```python
from build123d import *

# Parameters (mm, degrees)
EXTRUDE_1_DEPTH             = 2
EXTRUDE_2_REACH             = 86.23
EXTRUDE_2_DIRECTION_2_REACH = 86.23
CUT_EXTRUDE_2_DEPTH         = 114.341574455
FILLET_2_R                  = 1
SKETCH_8_R                  = 1.6
CUT_EXTRUDE_3_DEPTH         = 121.450189292
SKETCH_10_R                 = 1.6
SKETCH_10_W                 = 3.5
SKETCH_10_H                 = 20
CUT_EXTRUDE_5_DEPTH         = 86.056598939
SKETCH_11_R                 = 8.05
SKETCH_11_R_2               = 6.05
CUT_EXTRUDE_6_DEPTH         = 86.056598939
SKETCH_12_W                 = 25
SKETCH_12_H                 = 25
CUT_EXTRUDE_7_DEPTH         = 86.056598939
FILLET_3_R                  = 1


with BuildPart() as part:
    # 草图1 → 凸台-拉伸1 (new body)
    with BuildSketch(Plane.XY):
        with BuildLine():
            Line((72.25, -38.25), (72.25, 38.25))
            ThreePointArc((72.25, 38.25), (70.785533906, 41.785533906), (67.25, 43.25))
            Line((67.25, 43.25), (-67.25, 43.25))
            ThreePointArc((-67.25, 43.25), (-70.785533906, 41.785533906), (-72.25, 38.25))
            Line((-72.25, 38.25), (-72.25, -38.25))
            ThreePointArc((-72.25, -38.25), (-70.785533906, -41.785533906), (-67.25, -43.25))
            Line((-67.25, -43.25), (67.25, -43.25))
            ThreePointArc((67.25, -43.25), (70.785533906, -41.785533906), (72.25, -38.25))
        make_face()
    extrude(amount=EXTRUDE_1_DEPTH)

    # 凸台-拉伸2: up to this face of the body (flat: up to its plane)
    extrude_2_end = Plane(part.part.faces().sort_by_distance((0, 43.25, 1))[0])
    # 草图3 → 凸台-拉伸2 (add, up to the picked face)
    with BuildSketch(Plane(origin=(0, 0, 0), x_dir=(1, 0, 0), z_dir=(0, 1, 0)), mode=Mode.PRIVATE) as extrude_2_sk1:
        with BuildLine():
            Line((55.417603026, 0), (55.417603026, -2))
            ThreePointArc((55.417603026, -2), (64.361874936, -4.733500839), (70.25, -12))
            Line((70.25, -12), (72.25, -12))
            Line((72.25, -12), (72.25, -11.622664185))
            ThreePointArc((72.25, -11.622664185), (65.645211625, -3.187977102), (55.417603026, 0))
        make_face()
    extrude_2_tool1 = split(extrude(extrude_2_sk1.sketch, amount=EXTRUDE_2_REACH, mode=Mode.PRIVATE), bisect_by=extrude_2_end, keep=Keep.BOTH, mode=Mode.PRIVATE)
    add(extrude_2_tool1.solids().sort_by(Axis((64.519337, 0, 4.83454), (0, 1, 0)))[0])

    # 凸台-拉伸2 direction 2: up to this face of the body (flat: up to its plane)
    extrude_2_direction_2_end = Plane(part.part.faces().sort_by_distance((0, -43.25, 1))[0])
    # 草图3 → 凸台-拉伸2 direction 2 (add, up to the picked face)
    with BuildSketch(Plane(origin=(0, 0, 0), x_dir=(1, 0, 0), z_dir=(0, 1, 0)), mode=Mode.PRIVATE) as extrude_2_direction_2_sk1:
        with BuildLine():
            Line((55.417603026, 0), (55.417603026, -2))
            ThreePointArc((55.417603026, -2), (64.361874936, -4.733500839), (70.25, -12))
            Line((70.25, -12), (72.25, -12))
            Line((72.25, -12), (72.25, -11.622664185))
            ThreePointArc((72.25, -11.622664185), (65.645211625, -3.187977102), (55.417603026, 0))
        make_face()
    extrude_2_direction_2_tool1 = split(extrude(extrude_2_direction_2_sk1.sketch, amount=-EXTRUDE_2_DIRECTION_2_REACH, mode=Mode.PRIVATE), bisect_by=extrude_2_direction_2_end, keep=Keep.BOTH, mode=Mode.PRIVATE)
    add(extrude_2_direction_2_tool1.solids().sort_by(Axis((64.519337, 0, 4.83454), (0, -1, 0)))[0])

    # 草图6 → 切除-拉伸2 (cut, through all)
    with BuildSketch(Plane(origin=(0, 43.25, 0), x_dir=(1, 0, 0), z_dir=(0, 1, 0))):
        with BuildLine():
            Line((55.417603026, 0), (72.25, 0))
            Line((72.25, 0), (72.25, -2))
            Line((72.25, -2), (63.663814277, -2))
            ThreePointArc((63.663814277, -2), (59.660243713, -0.507144315), (55.417603026, 0))
        make_face()
    extrude(amount=-CUT_EXTRUDE_2_DEPTH, mode=Mode.SUBTRACT)

    # 圆角2
    fillet_2_edges = [part.edges().sort_by_distance(p)[0] for p in [
        (70.25, 0, 12),
    ]]
    fillet(fillet_2_edges, radius=FILLET_2_R)

    # 草图8 → 切除-拉伸3 (cut, through all)
    with BuildSketch(Plane(origin=(31.436723574, 0, -31.436723574), x_dir=(-0.7071067811865464, 0, -0.7071067811865488), z_dir=(0.7071067811865488, 0, -0.7071067811865464))):
        with Locations((-51.914084958, 6.5)):
            Circle(SKETCH_8_R)
        with Locations((-51.914084958, -6.5)):
            Circle(SKETCH_8_R)
    extrude(amount=-CUT_EXTRUDE_3_DEPTH, mode=Mode.SUBTRACT)

    # 草图10 → 切除-拉伸5 (cut, through all)
    with BuildSketch(Plane(origin=(0, 0, 0), x_dir=(-1, 0, 0), z_dir=(0, 0, -1))):
        with Locations(Location((65.1, 6, 0), (0, 0, 90))):
            Circle(SKETCH_10_R)
        with Locations(Location((65.1, -6, 0), (0, 0, 90))):
            Circle(SKETCH_10_R)
        with Locations((70.5, 0)):
            Rectangle(SKETCH_10_W, SKETCH_10_H)
    extrude(amount=-CUT_EXTRUDE_5_DEPTH, mode=Mode.SUBTRACT)

    # 草图11 → 切除-拉伸6 (cut, through all)
    with BuildSketch(Plane(origin=(0, 0, 0), x_dir=(-1, 0, 0), z_dir=(0, 0, -1))):
        with Locations((-47, 12.5)):
            Circle(SKETCH_11_R)
        with Locations((-47, -12.5)):
            Circle(SKETCH_11_R_2)
    extrude(amount=-CUT_EXTRUDE_6_DEPTH, mode=Mode.SUBTRACT)

    # 草图12 → 切除-拉伸7 (cut, through all)
    with BuildSketch(Plane(origin=(0, 0, 0), x_dir=(-1, 0, 0), z_dir=(0, 0, -1))):
        with Locations((-19.5, 20)):
            Rectangle(SKETCH_12_W, SKETCH_12_H)
    extrude(amount=-CUT_EXTRUDE_7_DEPTH, mode=Mode.SUBTRACT)

    # 圆角3
    fillet_3_edges = [part.edges().sort_by_distance(p)[0] for p in [
        (-72.25, 10, 1),
        (-72.25, -10, 1),
        (-68.75, -10, 1),
        (-68.75, 10, 1),
        (7, 32.5, 1),
        (7, 7.5, 1),
        (32, 7.5, 1),
        (32, 32.5, 1),
    ]]
    fillet(fillet_3_edges, radius=FILLET_3_R)


solid = part.part
```
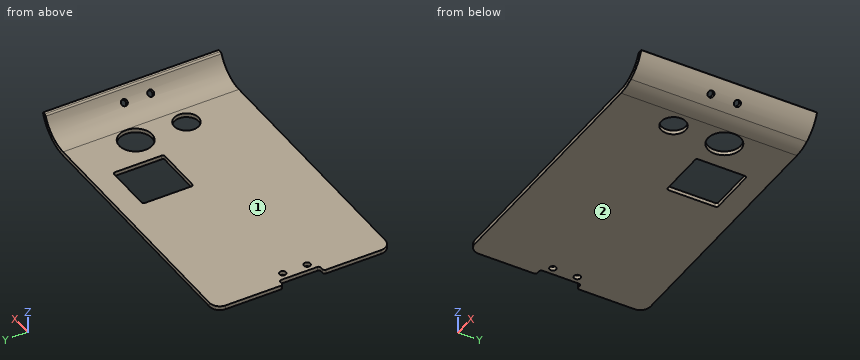
Design review of the part built by this model. Coordinates are the model's own, in mm. Face numbers are marked on the shaded views. A direction names the side the tool comes from. Coordinates: 2 decimals unless noted, no trailing zeros. Loops run counter-clockwise (first coordinate to the right, second up) from the corner with the lowest first, then second, coordinate; pieces in that order, holes last.
Q1. We need section D-D on y = -25.5. State the section outline as (x, z) points.
Reported:
outline: (-72.25, 0) - (55.42, 0) arc R18 ccw to (72.25, 11.62) - (72.25, 12) - (70.91, 12) arc R1 ccw to (70, 11.41) arc R16 cw to (55.42, 2) - (-72.25, 2) - close
Q2. We need section C-C on x = 16. State the section outline as (y, z) points, and give its area (3 significant figures).
Reported:
outline: (-43.25, 0) - (7.5, 0) - (7.5, 2) - (-43.25, 2) - close; (32.5, 0) - (43.25, 0) - (43.25, 2) - (32.5, 2) - close
area: 123 mm2
Q3. Tool access review of the marked faces 1 and 2: name each direction out of +Z, -Z, +X, -X, +Y, -Y from which nothing blocks a thin tool from reaching the whole face with its end or side.
Reported:
face 1: +Z, -X, +Y, -Y
face 2: -Z, +X, -X, +Y, -Y
Q4. We need section A-A on x = 47. State the section outline as (y, z) points.
Reported:
outline: (-43.25, 0) - (-18.55, 0) - (-18.55, 2) - (-43.25, 2) - close; (-6.45, 0) - (4.45, 0) - (4.45, 2) - (-6.45, 2) - close; (20.55, 0) - (43.25, 0) - (43.25, 2) - (20.55, 2) - close
Q5. For pin 1 (4 mm diameter, centred on x = -65.1, y = 6, fed in from +Z); pin 2 (4 mm diameter, centred on y = -17.5, z = 9.5, fed in from -X); pin 3 (1.6 mm diameter, centred on y = 18.5, z = 0.5, fed in from +X), all flat-tipped, find the tip position at first contact; note any pin that passes through.
Reported:
pin 1: stops at z = 2
pin 2: stops at x = 67.49
pin 3: stops at x = 62.13
Q6. We need section B-B on y = 12.5. State the section outline as (x, z) points.
Reported:
outline: (-72.25, 0) - (7, 0) - (7, 2) - (-72.25, 2) - close; (32, 0) - (38.95, 0) - (38.95, 2) - (32, 2) - close; (55.05, 0) - (55.42, 0) arc R18 ccw to (72.25, 11.62) - (72.25, 12) - (70.91, 12) arc R1 ccw to (70, 11.41) arc R16 cw to (55.42, 2) - (55.05, 2) - close
Q7. To check wall thickness, follow line 1 (Y direction, x = -65.1, z = 1.25); line 2 (Y direction, x = 47, z = 1.35); line 3 (Z direction, x = -16, y = 17). State the ranges of each line that lie inside material, in increasing order.
Reported:
line 1: y = -43.25 to -7.6, -4.4 to 4.4, 7.6 to 43.25
line 2: y = -43.25 to -18.55, -6.45 to 4.45, 20.55 to 43.25
line 3: z = 0 to 2
